Part print with two shaded views. Sizes in mm from the minimum x, y, z corner. A direction names the side the tool comes from. Give positions to 0.01 mm unless a question says otherwise; leave off trailing zeros. Write each loop counter-clockwise with the first axis right and the second up, starting at its lowest first coordinate (ties: lowest second). Pieces come first, ordered by that corner, then holes.
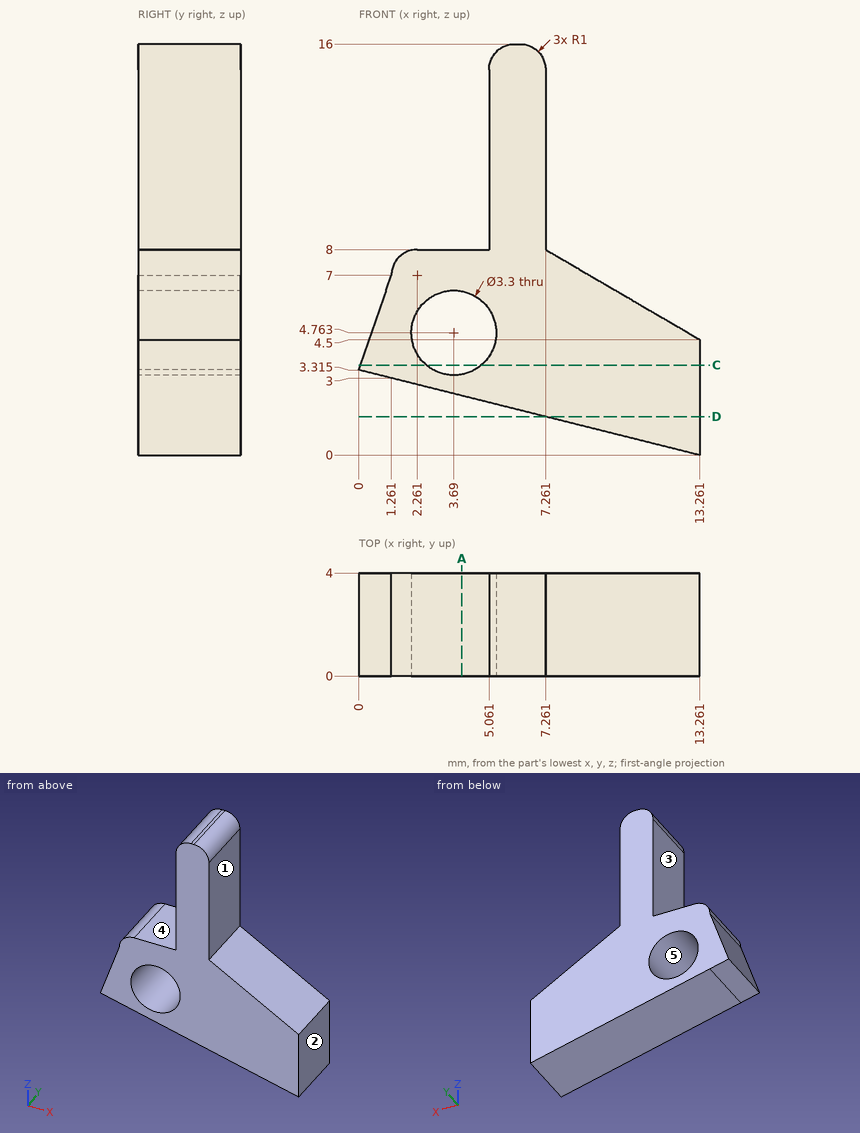
1) Mould opens along Z. For the marked faces 3, 4 and 5 say: +Z half, -Z half, draft (parallel to the pull), parting line (faces both ways), or undercut.
Check result:
face 3: draft
face 4: +Z half
face 5: undercut
2) Saw through at C-C (z = 3.5). Write the cut outline in (x, y), and give its area (3 significant figures).
Check result:
outline: (0.06, 0) - (2.63, 0) - (2.63, 4) - (0.06, 4) - close; (4.75, 0) - (13.26, 0) - (13.26, 4) - (4.75, 4) - close
area: 44.3 mm2
3) Saw through at D-D (z = 1.5). Write the cut outline in (x, y), and give its area (3 significant figures).
Check result:
outline: (7.26, 0) - (13.26, 0) - (13.26, 4) - (7.26, 4) - close
area: 24.0 mm2
4) 3-axis set-ups, long thin cutter, end or side, ignore diameter. For the marked faces 1 and 2: which of +Z, -Z, +X, -X, +Y, -Y reach the whole face in a straight line?
Check result:
face 1: +Z, +X, +Y, -Y
face 2: +Z, -Z, +X, +Y, -Y
5) Drill centre lines: L1, parallel to X at y = 3, z = 11; L2, parallel to X at y = 3.3, z = 5 (1 decimal); L3, parallel to Z at x = 2.5, y = 1.4 (1 decimal). Where is each one in solid material? Low to high.
Check result:
L1: x = 5.06 to 7.26
L2: x = 0.6 to 2.1, 5.3 to 12.4
L3: z = 2.7 to 3.6, 5.9 to 8
6) Flat gauge pins, fed straight in: P1, Ø0.8, axis at x = 3.5, y = 2, coming from the +Z side; P2, Ø2, axis at y = 2.5, z = 13, coming from the -X side; P3, Ø1, axis at y = 1, z = 6.5, coming from the +X side. Where does each tip first touch, or does it go through?
Check result:
P1: stops at z = 8
P2: stops at x = 5.06
P3: stops at x = 10.69
7) Saw through at A-A (x = 4). Write the cut outline in (y, z) (1 decimal).
Check result:
outline: (0, 2.3) - (4, 2.3) - (4, 3.1) - (0, 3.1) - close; (0, 6.4) - (4, 6.4) - (4, 8) - (0, 8) - close
